Build history of the part. All positions in model axes, mm. A direction names the side the tool comes from. Round coordinates to 2 decimals unless told otherwise and drop trailing zeros. Loops run counter-clockwise (first coordinate to the right, second up) from the corner with the lowest first, then second, coordinate; pieces in that order, holes last. Notation, with made-up numbers: (71.25, 87.5) -> (99.25, 87.5) arc R20 ccw to (99.25, 112.5) -> close; hole circle Ø4 at (31, 48.25). An arc over 180 degrees is marked (long way). Put each result on its own line as item: value. Start each with the question number.
Item 1: Cut at C-C, the plane y = -28. List the corners of the cut face in (x, z).
Item 2: Cut at B-B, the plane x = 1052.5. List the corners of the cut face in (y, z).
Item 3: Tool access for faces 1 (the flat face through (753, -17, 29)), 2 (the flat face through (753, 0, 20)): list every direction of +Z, -Z, +X, -X, +Y, -Y with a clear straight run to the whole face (end or side of a thin tool).
Item 4: Flat gauge pins, fed straight in: pin 1 Ø6 at (x, y) = (697, -21.5) entering from +Z; pin 2 Ø8 at (y, z) = (-35, 14) entering from -X; pin 3 Ø10 at (y, z) = (-7.5, 33) entering from +X; pin 4 Ø1 at (y, z) = (-23.5, 19) entering from +X. Where does each tip first touch, or does it go through?
Item 5: Drill centre lines: probe 1 along Y at (x, z) = (466, 30); probe 2 along Z at (x, y) = (815, -34); probe 3 along X at (y, z) = (-17, 11.5). Where is each one in solid material? Low to high. Write a range as [from, to].
Item 6: Cut at A-A, the plane z = 6.5. List the corners of the cut face in (x, y), plus the area to 3 significant figures.
```python
from build123d import *

# Parameters (mm, degrees)
BOSS_EXTRU_1_DEPTH      = 1527
ENL_V_MAT_EXTRU_1_DEPTH = 41
ENL_V_MAT_EXTRU_2_DEPTH = 41


with BuildPart() as part:
    # Esquisse1 → Boss.-Extru.1 (new body)
    with BuildSketch(Plane(origin=(0, 0, 0), x_dir=(0, 0, -1), z_dir=(1, 0, 0))):
        Polygon((0, 0), (-40, 0), (-40, -17), (-17, -17), (-17, -40), (0, -40), align=None)
    extrude(amount=BOSS_EXTRU_1_DEPTH)

    # Esquisse2 → Enlèv. mat.-Extru.1 (cut, through all)
    with BuildSketch(Plane(origin=(0, 0, 0), x_dir=(1, 0, 0), z_dir=(0, 1, 0))):
        Polygon((1527, 0), (1487, -40), (1527, -40), align=None)
        Polygon((0, 0), (0, -40), (40, -40), align=None)
    extrude(amount=-ENL_V_MAT_EXTRU_1_DEPTH, mode=Mode.SUBTRACT)

    # Esquisse3 → Enlèv. mat.-Extru.2 (cut, through all)
    with BuildSketch(Plane(origin=(0, 0, 0), x_dir=(-1, 0, 0), z_dir=(0, 0, -1))):
        Polygon((-1527, 0), (-1487, -40), (-1527, -40), align=None)
        Polygon((-40, -40), (0, -40), (0, 0), align=None)
    extrude(amount=-ENL_V_MAT_EXTRU_2_DEPTH, mode=Mode.SUBTRACT)


solid = part.part
```
Reply:
1. outline: (28, 0) -> (1499, 0) -> (1499, 17) -> (28, 17) -> close
2. outline: (-40, 0) -> (0, 0) -> (0, 40) -> (-17, 40) -> (-17, 17) -> (-40, 17) -> close
3. face 1: +Z, +X, -X, -Y
3. face 2: +Z, -Z, +X, -X, +Y
4. pin 1: stops at z = 17
4. pin 2: stops at x = 31
4. pin 3: stops at x = 1499
4. pin 4: passes through
5. probe 1: y = [-17, 0]
5. probe 2: z = [0, 17]
5. probe 3: x = [17, 1510]
6. outline: (6.5, -6.5) -> (40, -40) -> (1487, -40) -> (1520.5, -6.5) -> (1520.5, 0) -> (6.5, 0) -> close
6. area: 59,400 mm^2
